Part model, mm, in its own coordinate system. A direction names the side the tool comes from. Coordinates: 2 decimals unless noted, no trailing zeros. Order: outer loops, then holes, each group sorted by start corner. A loop starts at its lowest first (then second) coordinate and runs counter-clockwise, first axis right, second up.
from build123d import *

# Parameters (mm, degrees)
SKETCH1_R           = 82.55
SKETCH1_R_2         = 2.54
SKETCH1_W           = 25.4
SKETCH1_H           = 2.54
SKETCH1_W_2         = 2.54
SKETCH1_H_2         = 25.4
BOSS_EXTRUDE1_DEPTH = 5.08


with BuildPart() as part:
    # Sketch1 → Boss-Extrude1 (new body)
    with BuildSketch(Plane(origin=(0, 0, 0), x_dir=(1, 0, 0), z_dir=(0, 1, 0))):
        with Locations(Location((0, 0, 0), (0, 0, 270))):
            Circle(SKETCH1_R)
        with Locations(Location((0, 0, 0), (0, 0, 270))):
            Circle(SKETCH1_R_2, mode=Mode.SUBTRACT)
        with Locations((64.77, 0)):
            Rectangle(SKETCH1_W, SKETCH1_H, mode=Mode.SUBTRACT)
        with Locations((0, 64.77)):
            Rectangle(SKETCH1_W_2, SKETCH1_H_2, mode=Mode.SUBTRACT)
        with Locations((0, -64.77)):
            Rectangle(SKETCH1_W_2, SKETCH1_H_2, mode=Mode.SUBTRACT)
        with Locations((-64.77, 0)):
            Rectangle(SKETCH1_W, SKETCH1_H, mode=Mode.SUBTRACT)
    extrude(amount=BOSS_EXTRUDE1_DEPTH)


solid = part.part
Q1. Wall check: line 1 along X through (y, z) = (2, 0); line 2 along X through (y, z) = (4.7, -68); line 3 along Z through (x, y) = (54.5, 1.9). Give the ranges that are in metal, low to high.
Results list:
line 1: x = -82.55 to -77.47, -52.07 to -2.54, 2.54 to 52.07, 77.47 to 82.55
line 2: x = -46.8 to -1.27, 1.27 to 46.8
line 3: z = -62 to -1.27, 1.27 to 62
Q2. Pin check, flat tips, straight feed: pin 1 Ø1.5 at (x, y) = (36.5, 3.5) entering from +Z; pin 2 Ø1.5 at (y, z) = (1, -20) entering from -X; pin 3 Ø1.5 at (x, y) = (-60, 2) entering from -Z. Stop position of each tip, or through.
Results list:
pin 1: stops at z = 74.41
pin 2: stops at x = -80.27
pin 3: stops at z = -57.48
Q3. Mould opens along Z. For faces 3 (the face through (-1.27, 3, -65)), 4 (the face through (81.848, 2.504, -10.746)), 5 (the face through (-17, 5.08, -1)) say: pulls with the +Z half, pulls with the -Z half, needs draft (parallel to the pull), parting line crosses it, or undercut.
Results list:
face 3: undercut
face 4: parting line crosses it
face 5: needs draft
Q4. Cut at B-B on x = 55.5. Write the cut outline in (y, z), and give its area (3 significant figures).
Results list:
outline: (0, -61.11) - (5.08, -61.11) - (5.08, -1.27) - (0, -1.27) - close; (0, 1.27) - (5.08, 1.27) - (5.08, 61.11) - (0, 61.11) - close
area: 608 mm2
Q5. Cut at C-C on z = -55.5. Write the cut outline in (x, y), and give its area (3 significant figures).
Results list:
outline: (-61.11, 0) - (-1.27, 0) - (-1.27, 5.08) - (-61.11, 5.08) - close; (1.27, 0) - (61.11, 0) - (61.11, 5.08) - (1.27, 5.08) - close
area: 608 mm2
Q6. Which spindle directions (+Z, -Z, +X, -X, +Y, -Y) get a long thin tool onto all of the face, cutting with end or side? Do faces 1 (the face through (1.27, 3, 65)), 2 (the face through (-17, 0, -1)). Say none if no direction does.
Results list:
face 1: +Y, -Y
face 2: +Z, -Z, +X, -X, -Y
Q7. Cut at A-A on y = 1. Write the cut outline in (x, z).
Results list:
outline: circle Ø165.1 at (0, 0); hole (-77.47, -1.27) - (-52.07, -1.27) - (-52.07, 1.27) - (-77.47, 1.27) - close; hole circle Ø5.08 at (0, 0); hole (-1.27, -77.47) - (1.27, -77.47) - (1.27, -52.07) - (-1.27, -52.07) - close; hole (-1.27, 52.07) - (1.27, 52.07) - (1.27, 77.47) - (-1.27, 77.47) - close; hole (52.07, -1.27) - (77.47, -1.27) - (77.47, 1.27) - (52.07, 1.27) - close
Q8. Cut at D-D on x = 17. Write the cut outline in (y, z).
Results list:
outline: (0, -80.78) - (5.08, -80.78) - (5.08, 80.78) - (0, 80.78) - close
